from build123d import *

# Parameters (mm, degrees)
F0_W     = 10.9982
F0_H     = 7.493
F0_W_2   = 8.001
F0_H_2   = 5.0038
F0_R     = 2.4892
F0_R_2   = 5.0038
F1_DEPTH = 5
F0_W_3   = 50
F0_H_3   = 22.5
F2_DEPTH = 5


with BuildPart() as f1:
    # F0 (on Front) → F1 (new body)
    with BuildSketch(Plane.XZ):
        with BuildLine():
            Line((32.930795, 54.273571), (-32.067805, 54.273571))
            Line((-32.067805, 54.273571), (-32.067805, -39.597668))
            ThreePointArc((-32.067805, -39.597668), (-30.322229, -43.811862), (-26.108036, -45.557438))
            Line((-26.108036, -45.557438), (26.971026, -45.557438))
            ThreePointArc((26.971026, -45.557438), (31.185219, -43.811862), (32.930795, -39.597668))
            Line((32.930795, -39.597668), (32.930795, 54.273571))
        make_face()
        Polygon((-24.558977, -43.883898), (-30.058077, -43.883898), (-30.058077, -36.390898), (-19.059877, -36.390898), (-19.059877, -43.883898), align=None, mode=Mode.SUBTRACT)
        Polygon((-24.497674, -31.799856), (-29.996774, -31.799856), (-29.996774, -24.306856), (-18.998574, -24.306856), (-18.998574, -31.799856), align=None, mode=Mode.SUBTRACT)
        Polygon((-24.558977, -19.887637), (-30.058077, -19.887637), (-30.058077, -12.394637), (-19.059877, -12.394637), (-19.059877, -19.887637), align=None, mode=Mode.SUBTRACT)
        Polygon((-11.717032, -43.883901), (-17.216132, -43.883901), (-17.216132, -36.390901), (-6.217932, -36.390901), (-6.217932, -43.883901), align=None, mode=Mode.SUBTRACT)
        Polygon((-11.655728, -31.799859), (-17.154828, -31.799859), (-17.154828, -24.306859), (-6.156628, -24.306859), (-6.156628, -31.799859), align=None, mode=Mode.SUBTRACT)
        Polygon((-11.717032, -19.887639), (-17.216132, -19.887639), (-17.216132, -12.394639), (-6.217932, -12.394639), (-6.217932, -19.887639), align=None, mode=Mode.SUBTRACT)
        Polygon((-24.497674, -7.803595), (-29.996774, -7.803595), (-29.996774, -0.310595), (-18.998574, -0.310595), (-18.998574, -7.803595), align=None, mode=Mode.SUBTRACT)
        Polygon((-27.643991, 5.020094), (-29.990563, 5.020094), (-29.990563, 10.023894), (-21.989563, 10.023894), (-21.989563, 5.020094), align=None, mode=Mode.SUBTRACT)
        Polygon((-26.28431, 14.722894), (-29.987015, 14.722894), (-29.987015, 19.726694), (-21.987015, 19.726694), (-21.987015, 14.722894), align=None, mode=Mode.SUBTRACT)
        Polygon((-25.983574, 24.419945), (-29.996774, 24.419945), (-29.996774, 29.423745), (-21.995774, 29.423745), (-21.995774, 24.419945), align=None, mode=Mode.SUBTRACT)
        Polygon((-11.655728, -7.803598), (-17.154828, -7.803598), (-17.154828, -0.310598), (-6.156628, -0.310598), (-6.156628, -7.803598), align=None, mode=Mode.SUBTRACT)
        Polygon((-17.148439, 5.016294), (-19.500365, 5.016294), (-19.500365, 10.020094), (-11.499365, 10.020094), (-11.499365, 5.016294), align=None, mode=Mode.SUBTRACT)
        Polygon((-7.183166, 5.020094), (-9.010165, 5.020094), (-9.010165, 10.020094), (-1.009165, 10.020094), (-1.009165, 5.020094), align=None, mode=Mode.SUBTRACT)
        Polygon((-15.484615, 14.722894), (-19.497815, 14.722894), (-19.497815, 19.726694), (-11.496815, 19.726694), (-11.496815, 14.722894), align=None, mode=Mode.SUBTRACT)
        Polygon((-15.493374, 24.419945), (-19.506574, 24.419945), (-19.506574, 29.423745), (-11.505574, 29.423745), (-11.505574, 24.419945), align=None, mode=Mode.SUBTRACT)
        Polygon((-5.823485, 14.722894), (-9.007615, 14.722894), (-9.007615, 19.726694), (-1.006615, 19.726694), (-1.006615, 14.722894), align=None, mode=Mode.SUBTRACT)
        Polygon((-5.52275, 24.419945), (-9.016374, 24.419945), (-9.016374, 29.423745), (-1.015374, 29.423745), (-1.015374, 24.419945), align=None, mode=Mode.SUBTRACT)
        Polygon((1.135368, -43.883901), (-4.363732, -43.883901), (-4.363732, -36.390901), (6.634468, -36.390901), (6.634468, -43.883901), align=None, mode=Mode.SUBTRACT)
        Polygon((1.196672, -31.799859), (-4.302428, -31.799859), (-4.302428, -24.306859), (6.695772, -24.306859), (6.695772, -31.799859), align=None, mode=Mode.SUBTRACT)
        Polygon((14.020374, -43.883901), (8.521274, -43.883901), (8.521274, -36.390901), (19.519474, -36.390901), (19.519474, -43.883901), align=None, mode=Mode.SUBTRACT)
        with Locations((14.020374, -28.053359)):
            Rectangle(F0_W, F0_H, mode=Mode.SUBTRACT)
        Polygon((1.135368, -19.887639), (-4.363732, -19.887639), (-4.363732, -12.394639), (6.634468, -12.394639), (6.634468, -19.887639), align=None, mode=Mode.SUBTRACT)
        Polygon((14.020374, -19.887639), (8.521274, -19.887639), (8.521274, -12.394639), (19.519474, -12.394639), (19.519474, -19.887639), align=None, mode=Mode.SUBTRACT)
        Polygon((25.782729, -43.883901), (21.115824, -43.883901), (21.115824, -36.390901), (31.015452, -36.390901), (31.015452, -43.883901), align=None, mode=Mode.SUBTRACT)
        Polygon((25.844033, -31.799859), (21.177127, -31.799859), (21.177127, -24.306859), (31.076756, -24.306859), (31.076756, -31.799859), align=None, mode=Mode.SUBTRACT)
        Polygon((25.782729, -19.887639), (21.115824, -19.887639), (21.115824, -12.394639), (31.015452, -12.394639), (31.015452, -19.887639), align=None, mode=Mode.SUBTRACT)
        Polygon((1.196672, -7.803598), (-4.302428, -7.803598), (-4.302428, -0.310598), (6.695772, -0.310598), (6.695772, -7.803598), align=None, mode=Mode.SUBTRACT)
        with Locations((5.480535, 7.521994)):
            Rectangle(F0_W_2, F0_H_2, mode=Mode.SUBTRACT)
        Polygon((14.081677, -7.803598), (8.582577, -7.803598), (8.582577, -0.310598), (19.580777, -0.310598), (19.580777, -7.803598), align=None, mode=Mode.SUBTRACT)
        Polygon((12.818122, 5.020094), (11.970235, 5.020094), (11.970235, 10.006707), (19.971235, 10.006707), (19.971235, 5.020094), align=None, mode=Mode.SUBTRACT)
        with Locations((5.483085, 17.224794)):
            Rectangle(F0_W_2, F0_H_2, mode=Mode.SUBTRACT)
        Polygon((9.474826, 24.419945), (1.473826, 24.419945), (1.473826, 29.423745), (9.474826, 29.423745), (9.474826, 26.934545), align=None, mode=Mode.SUBTRACT)
        Polygon((14.177803, 14.722894), (11.972785, 14.722894), (11.972785, 19.726694), (19.972785, 19.726694), (19.972785, 14.722894), align=None, mode=Mode.SUBTRACT)
        Polygon((14.478539, 24.419945), (11.964026, 24.419945), (11.964026, 29.423745), (19.965026, 29.423745), (19.965026, 24.419945), align=None, mode=Mode.SUBTRACT)
        Polygon((25.844033, -7.803598), (21.177127, -7.803598), (21.177127, -0.310598), (31.076756, -0.310598), (31.076756, -7.803598), align=None, mode=Mode.SUBTRACT)
        Polygon((24.846989, 5.002907), (22.460435, 5.002907), (22.460435, 10.006707), (30.797195, 10.006707), (30.797195, 5.002907), align=None, mode=Mode.SUBTRACT)
        Polygon((26.16669, 14.722894), (22.461985, 14.722894), (22.461985, 19.726694), (30.801985, 19.726694), (30.801985, 14.722894), align=None, mode=Mode.SUBTRACT)
        Polygon((26.467426, 24.419945), (22.454226, 24.419945), (22.454226, 29.423745), (30.796636, 29.423745), (30.796636, 24.419945), align=None, mode=Mode.SUBTRACT)
        Polygon((-25.983574, 34.27997), (-29.996351, 34.27997), (-29.996351, 39.453434), (-21.995774, 39.453434), (-21.995774, 34.27997), align=None, mode=Mode.SUBTRACT)
        with Locations((-25.996883, 48.632245)):
            Circle(F0_R, mode=Mode.SUBTRACT)
        Polygon((-15.493374, 34.279969), (-19.506574, 34.279969), (-19.506574, 39.283769), (-11.505574, 39.283769), (-11.505574, 34.279969), align=None, mode=Mode.SUBTRACT)
        with Locations((-15.493563, 48.632245)):
            Circle(F0_R, mode=Mode.SUBTRACT)
        with Locations((0.229226, 43.927145)):
            Circle(F0_R_2, mode=Mode.SUBTRACT)
        Polygon((14.478539, 34.27997), (11.964026, 34.27997), (11.964026, 39.28377), (19.965026, 39.28377), (19.965026, 34.27997), (15.964526, 34.27997), align=None, mode=Mode.SUBTRACT)
        with Locations((15.964526, 48.632245)):
            Circle(F0_R, mode=Mode.SUBTRACT)
        Polygon((26.467426, 34.449634), (22.454226, 34.449634), (22.454226, 39.453434), (30.796636, 39.453434), (30.796636, 34.449634), align=None, mode=Mode.SUBTRACT)
        with Locations((26.467426, 48.632245)):
            Circle(F0_R, mode=Mode.SUBTRACT)
    extrude(amount=F1_DEPTH)

    # F0 (on Front) → F2 (join)
    with BuildSketch(Plane.XZ):
        with BuildLine():
            Line((-32.067805, 103.682429), (-32.067805, 54.273571))
            Line((-32.067805, 54.273571), (32.930795, 54.273571))
            Line((32.930795, 54.273571), (32.930795, 103.682429))
            ThreePointArc((32.930795, 103.682429), (31.243691, 107.755458), (27.170661, 109.442562))
            Line((27.170661, 109.442562), (-26.307672, 109.442562))
            ThreePointArc((-26.307672, 109.442562), (-30.380701, 107.755458), (-32.067805, 103.682429))
        make_face()
        with Locations((-0.495507, 80.151956)):
            Rectangle(F0_W_3, F0_H_3, mode=Mode.SUBTRACT)
    extrude(amount=F2_DEPTH)


solid = f1.part
Design review of the part built by this model. Coordinates are the model's own, in mm. Round coordinates to 2 decimals unless told otherwise and drop trailing zeros. Loops run counter-clockwise (first coordinate to the right, second up) from the corner with the lowest first, then second, coordinate; pieces in that order, holes last. Notation, with made-up numbers: M 14.5,-35.75 L 41.5,-35.75 A25 ccw 41.5,-13.75 Z; hole C 75.5,2.5 d4. An arc over 180 degrees is marked long. Answer as a JSON object with one key per item and string values.
Item 1: We need section C-C on y = -1.5. State how many separate pieces and enclosed holes the cut face has, and give its area (3 significant figures).
Answer sheet:
{"separate pieces": "1", "enclosed holes": "48", "area": "6,260 mm^2"}
Item 2: We need section B-B on z = 73. Give the boundary of the cut face in (x, y).
Answer sheet:
{"outline": "M -32.07,-5 L -25.5,-5 L -25.5,0 L -32.07,0 Z; M 24.5,-5 L 32.93,-5 L 32.93,0 L 24.5,0 Z"}
Item 3: We need section A-A on z = 27. Give the boundary of the cut face in (x, y).
Answer sheet:
{"outline": "M -32.07,-5 L -30,-5 L -30,0 L -32.07,0 Z; M -22,-5 L -19.51,-5 L -19.51,0 L -22,0 Z; M -11.51,-5 L -9.02,-5 L -9.02,0 L -11.51,0 Z; M -1.02,-5 L 1.47,-5 L 1.47,0 L -1.02,0 Z; M 9.47,-5 L 11.96,-5 L 11.96,0 L 9.47,0 Z; M 19.97,-5 L 22.45,-5 L 22.45,0 L 19.97,0 Z; M 30.8,-5 L 32.93,-5 L 32.93,0 L 30.8,0 Z"}
Item 4: Wall thickness on L1, parallel to X at y = -4.25, z = 34.5; L2, parallel to X at y = -2.3, z = -26; L3, parallel to X at y = -0.65, z = 70.5: over which ranges is each line inside the solid? List them lowest first. Write a range as from..to.
Answer sheet:
{"L1": "x = -32.07..-30, -22..-19.51, -11.51..11.96, 19.97..22.45, 30.8..32.93", "L2": "x = -32.07..-30, -19..-17.15, -6.16..-4.3, 6.7..8.52, 19.52..21.18, 31.08..32.93", "L3": "x = -32.07..-25.5, 24.5..32.93"}
